Verification items for the finished model (mm, model axes). A direction names the side the tool comes from. Give positions to 0.01 mm unless a question says otherwise; leave off trailing zeros. Answer as a JSON object with one key per item and string values.
Autodesk Inventor part; units mm, degrees
ref_plane "YZ Plane" through (0, 0, 0) normal (1, 0, 0) x (0, 1, 0)
ref_plane "XZ Plane" through (0, 0, 0) normal (0, 1, 0) x (-1, 0, 0)
ref_plane "XY Plane" through (0, 0, 0) normal (0, 0, 1) x (1, 0, 0)
sketch "Sketch1" plane through (0, 0, 0) normal (0, 1, 0) x (-1, 0, 0)
  circle A0 centre (0, 0) radius 34.925
  dimension "d0" = 69.85
extrude "Extrusion1" add sketch "Sketch1" along normal blind 12.7
sketch "Sketch2" plane through (0, 12.7, 0) normal (0, 1, 0) x (1, 0, 0)
  circle A0 centre (0, 0) radius 17.78
  circle A1 centre (0, 0) radius 19.05
  circle A2 centre (0, 0) radius 21.59
  circle A3 centre (0, 0) radius 24.13
  dimension "d3" = 35.56
  dimension "d4" = 38.1
  dimension "d5" = 43.18
  dimension "d6" = 48.26
extrude "Extrusion2" cut sketch "Sketch2" against normal blind 1.27 contours A3
extrude "Extrusion3" cut sketch "Sketch2" against normal blind 1.778 contours A2
extrude "Extrusion4" cut sketch "Sketch2" against normal blind 2.286 contours A1
sketch "Sketch3" plane through (0, 0, 0) normal (0, -1, 0) x (1, 0, 0)
  circle A0 centre (0, 0) radius 19.05
  circle A1 centre (0, 0) radius 21.59
  circle A2 centre (0, 0) radius 24.13
sketch "Sketch4" plane through (0, 0, 0) normal (0, -1, 0) x (1, 0, 0)
  circle A0 centre (0, 0) radius 17.78
  circle A1 centre (0, 0) radius 19.05
extrude "Extrusion5" cut sketch "Sketch3" against normal blind 1.27 contours A2
extrude "Extrusion6" cut sketch "Sketch3" against normal blind 1.778 contours A1
extrude "Extrusion7" cut sketch "Sketch4" against normal blind 2.286
chamfer "Chamfer1" distance 1.27 angle 45 2 edges at (34.925, 12.7, 0) (34.925, 0, 0)
sketch "Sketch5" plane through (0, 12.7, 0) normal (0, 1, 0) x (1, 0, 0)
  point P0 (0, 0)
sketch "Sketch6" plane through (0, 12.7, 0) normal (0, 1, 0) x (1, 0, 0)
  point P0 (0, 0)
sketch "Sketch7" plane through (0, 12.7, 0) normal (0, 1, 0) x (1, 0, 0)
  line L0 (0, 0) -> (-29.3624, 0)
  dimension "d22" = 29.3624
hole "Hole1" at (-29.3624, 12.7, 0) direction (0, -1, 0) diameter 5.4102 end through all
chamfer "Chamfer2" distance 0.254 angle 45 1 edges at (-29.3624, 12.7, -2.7051)
chamfer "Chamfer3" distance 0.254 angle 45 1 edges at (-29.3624, 0, -2.7051)
pattern_circular "Circular Pattern1" count 6 over 360 about axis through (0, 12.7, 0) along (0, -1, 0) of "Hole1", "Chamfer2"
sketch "Sketch8" plane through (0, 12.7, 0) normal (0, 1, 0) x (1, 0, 0)
  line L0 (0, 0) -> (0.7937, 0)
  line L1 (0.7937, 0) -> (0.7937, 24.1169)
  circle A0 centre (0, 0) radius 24.13
  circle A1 centre (0, 0) radius 34.925
  line L2 (0.7937, 34.916) -> (0.7937, 24.1169)
  line L3 (0.7937, 0) -> (-0.7937, 0)
  line L4 (-0.7937, 0) -> (-0.7937, 34.916)
  line L5 (-0.7937, 34.916) -> (0.7937, 34.916)
  line L6 (0.7937, 5.7639) -> (0.7937, -35.1013)
  line L7 (0.7937, -35.1013) -> (-0.7937, -35.1013)
  line L8 (-0.7937, -35.1013) -> (-0.7937, 0)
  line L9 (-0.7937, -24.0567) -> (0.7937, -24.0567)
  line L10 (0.7937, 24.1169) -> (-0.7937, 24.1169)
  point P0 (-0.7937, -24.1169)
  point P1 (-0.7938, -34.916)
  point P2 (0.7937, -34.916)
  point P3 (0.7938, -24.1169)
  point P4 (-0.7937, 24.1169)
  dimension "d39" = 0.7937
  dimension "d40" = 1.5875
extrude "Extrusion8" cut sketch "Sketch8" against normal blind 1.27 contours L4 L5 L2 A0 | L6 A1 L8 A0
hole "Hole2" at (0, 12.7, 0) direction (0, -1, 0) diameter 10.9982 end through all
sketch "Sketch9" plane through (0, 12.7, 0) normal (0, 1, 0) x (1, 0, 0)
  line L0 (0, 0) -> (13.6144, 0)
  dimension "d50" = 13.6144
hole "Hole3" at (13.6144, 12.7, 0) direction (0, -1, 0) diameter 4.9022 end through all
pattern_circular "Circular Pattern2" count 3 over 360 about axis through (0, -86.8959, 0) along (0, 1, 0) of "Hole3"
properties part number "2.75 flange"
(1) Release check for a two-part mould opening along Z. For faces 1 (the cylindrical face through (27.715, 6.279, 21.251)), 2 (the flat face through (-7, 11.43, 21)), 3 (the flat face through (-24.5, 12.7, -2.3)) record: pulls with the +Z half, pulls with the -Z half, needs draft (parallel to the pull), parting line crosses it, or undercut.
Computed values:
{"face 1": "parting line crosses it", "face 2": "undercut", "face 3": "needs draft"}
(2) Gauge pin test, flat ends, axial feed: pin 1 Ø4.5 at (x, z) = (-6.81, 11.79) entering from -Y; pin 2 Ø2 at (y, z) = (9.5, 11.5) entering from -X; pin 3 Ø1.5 at (x, z) = (12.5, 19.5) entering from -Y; pin 4 Ø2 at (y, z) = (10, 13.5) entering from +X. Record the tip position at first contact, or that the pin passes through.
Computed values:
{"pin 1": "passes through", "pin 2": "stops at x = -33.31", "pin 3": "stops at y = 1.27", "pin 4": "stops at x = 32.61"}
(3) Material ranges on line 1 along Z through (x, y) = (0, 2) (3 decimals); line 2 along X through (y, z) = (8.25, 0) (1 decimal); line 3 along X through (y, z) = (10.5, 15.5), recorded low to high. Write a range as [from, to].
Computed values:
{"line 1": "z = [-34.925, -19.05], [-17.78, -5.499], [5.499, 17.78], [19.05, 34.925]", "line 2": "x = [-34.9, -32.1], [-26.7, -5.5], [5.5, 11.2], [16.1, 26.7], [32.1, 34.9]", "line 3": "x = [-31.3, -11.07], [-8.71, 8.71], [11.07, 31.3]"}
(4) Section check A-A (z = 0). Count the separate pieces of the cut face and the enclosed holes in it, then the cut area to 3 significant figures.
Computed values:
{"separate pieces": "5", "enclosed holes": "0", "area": "502 mm²"}
(5) Access from +Z, -Z, +X, -X, +Y, -Y to the whole of each face (thin tool, end or side, straight path). Record for faces 4 (the cylindrical face through (-15.12, 10.67, 11.59)), 5 (the flat face through (-18, 1.27, -12.4)), 6 (the flat face through (25, 12.7, 0)).
Computed values:
{"face 4": "+Y", "face 5": "-Y", "face 6": "+Z, -Z, +X, -X, +Y"}
